For this review, use the dimensioned drawing (mm, ordinates from the lowest corner) and the shaded views. A direction names the side the tool comes from. Give positions to 0.01 mm unless a question says otherwise; leave off trailing zeros. Order: outer loops, then holes, each group sorted by start corner. A loop starts at its lowest first (then second) coordinate and runs counter-clockwise, first axis right, second up. Notation, with made-up numbers: (-1.5, 29.25) -> (19.5, 29.25) arc R21 ccw to (19.5, 57.25) -> close; hole circle Ø9 at (44.25, 52). An arc over 180 degrees is marked (long way). Return JSON: item names as keys, results as strings.
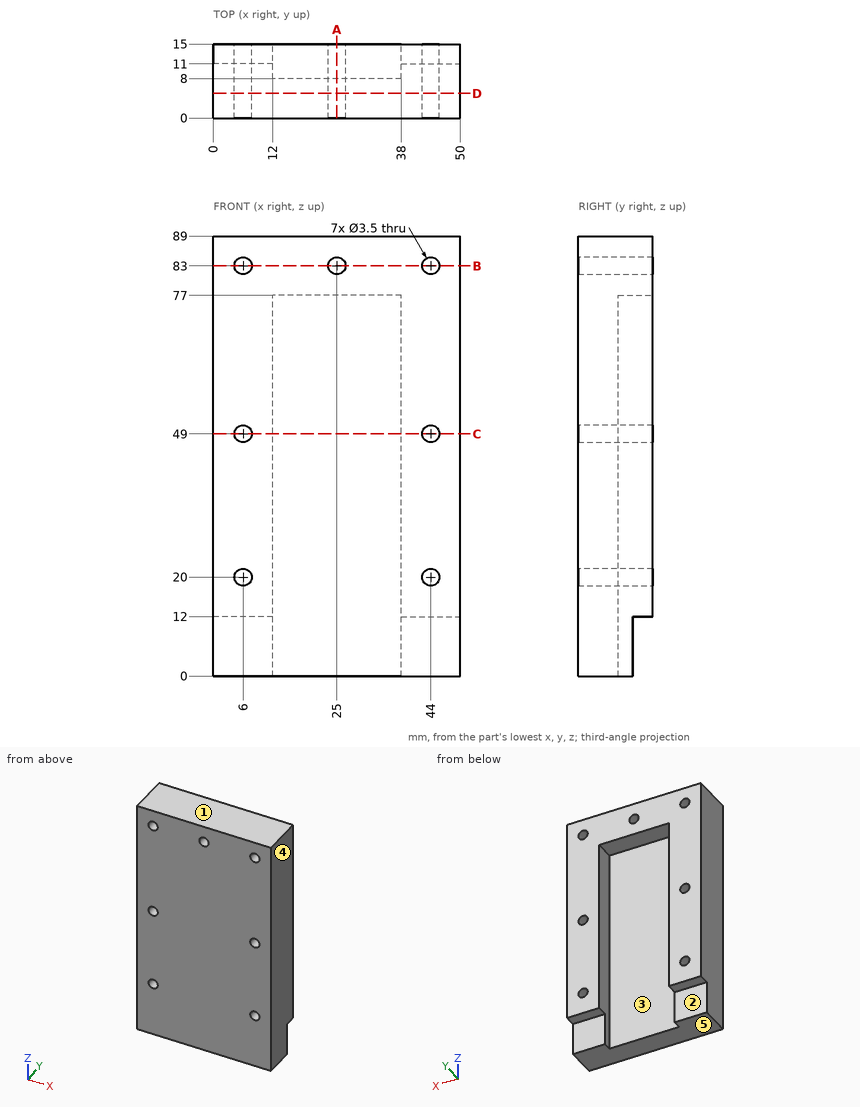
Item 1: Machinability: for the marked faces 1 and 2, which of the approach directions +Z, -Z, +X, -X, +Y, -Y give a long, thin tool a straight path to every point of the face, cutting with its end or side? Answer none if there is none.
Result set:
{"face 1": "+Z, +X, -X, +Y, -Y", "face 2": "-Z, +X, -X, +Y"}
Item 2: Wall thickness on L1, parallel to X at y = 8.5, z = 49; L2, parallel to X at y = 9.25, z = 83; L3, parallel to X at y = 10.25, z = 67: over which ranges is each line inside the solid? List them lowest first. Write a range as [from, to].
Result set:
{"L1": "x = [0, 4.25], [7.75, 12], [38, 42.25], [45.75, 50]", "L2": "x = [0, 4.25], [7.75, 23.25], [26.75, 42.25], [45.75, 50]", "L3": "x = [0, 12], [38, 50]"}
Item 3: Add section B-B (z = 83). Give the boundary of the cut face in (x, y), plus the area to 4 significant figures.
Result set:
{"outline": "(0, 0) -> (4.25, 0) -> (4.25, 15) -> (0, 15) -> close; (7.75, 0) -> (23.25, 0) -> (23.25, 15) -> (7.75, 15) -> close; (26.75, 0) -> (42.25, 0) -> (42.25, 15) -> (26.75, 15) -> close; (45.75, 0) -> (50, 0) -> (50, 15) -> (45.75, 15) -> close", "area": "592.5 mm^2"}
Item 4: Add section C-C (z = 49). Give the boundary of the cut face in (x, y), plus the area to 3 significant figures.
Result set:
{"outline": "(0, 0) -> (4.25, 0) -> (4.25, 15) -> (0, 15) -> close; (7.75, 0) -> (42.25, 0) -> (42.25, 15) -> (38, 15) -> (38, 8) -> (12, 8) -> (12, 15) -> (7.75, 15) -> close; (45.75, 0) -> (50, 0) -> (50, 15) -> (45.75, 15) -> close", "area": "463 mm^2"}
Item 5: Mouldability with a two-part tool opening along X and no side actions: class the marked faces 3, 4 and 5 as released by +X, released by -X, zero draft, split by the parting line, or undercut.
Result set:
{"face 3": "undercut", "face 4": "released by +X", "face 5": "zero draft"}
Item 6: For pin 1 (3.5 mm diameter, centred on x = 19, y = 12, fed in from -Z); pin 2 (3 mm diameter, centred on x = 46.5, y = 13.5, fed in from -Z); pin 3 (4.5 mm diameter, centred on x = 6, z = 49, fed in from -Y); pin 4 (1 mm diameter, centred on x = 35.5, z = 14.5, fed in from +Y), all flat-tipped, find the tip position at first contact; note any pin that passes through.
Result set:
{"pin 1": "stops at z = 77", "pin 2": "stops at z = 12", "pin 3": "stops at y = 0", "pin 4": "stops at y = 8"}
Item 7: Add section A-A (x = 25). Give the boundary of the cut face in (y, z), plus the area to 4 significant figures.
Result set:
{"outline": "(0, 0) -> (8, 0) -> (8, 77) -> (15, 77) -> (15, 81.25) -> (0, 81.25) -> close; (0, 84.75) -> (15, 84.75) -> (15, 89) -> (0, 89) -> close", "area": "743.5 mm^2"}
Item 8: Add section D-D (y = 5). Give the boundary of the cut face in (x, z).
Result set:
{"outline": "(0, 0) -> (50, 0) -> (50, 89) -> (0, 89) -> close; hole circle Ø3.5 at (6, 20); hole circle Ø3.5 at (6, 49); hole circle Ø3.5 at (6, 83); hole circle Ø3.5 at (25, 83); hole circle Ø3.5 at (44, 20); hole circle Ø3.5 at (44, 49); hole circle Ø3.5 at (44, 83)"}
